For this review, take the finished solid that the model builds, in its own axes (mm). A direction names the side the tool comes from. Coordinates: 2 decimals unless noted, no trailing zeros. Write each loop counter-clockwise with the first axis right and the second up, starting at its lowest first coordinate (ties: lowest second). Pieces come first, ordered by that corner, then holes.
1) For faces 4 (the face through (15, 8, 0)), 5 (the face through (30, -6.5, -0.2)), list the 3-axis set-ups (+Z, -Z, +X, -X, +Y, -Y) from which the entire face can be reached by the end or side of a thin tool; tool diameter is ignored.
2) To check wall thickness, follow line 1 along Y through (x, z) = (12, -3.25); line 2 along Y through (x, z) = (22, -2.25); line 3 along Z through (x, y) = (14, -1). State the ranges of each line that lie inside material, in increasing order.
3) Mouldability with a two-part tool opening along Y and no side actions: class faces 1 (the face through (15, 7, 2)), 2 (the face through (15.21, -7.17, -6.97)), 3 (the face through (0, -6.5, -0.2)) as pulls with the +Y half, pulls with the -Y half, needs draft (parallel to the pull), parting line crosses it, or undercut.
4) We need section D-D on z = -9.25. Write out the cut boundary in (x, y), then the cut area to 3 significant figures.
5) We need section B-B on y = -2.5. Write out the cut boundary in (x, z), then the cut area to 3 significant figures.
6) We need section A-A on x = 6.5. Write out the cut boundary in (y, z).
7) We need section C-C on z = 4.5. Write out the cut boundary in (x, y), then the cut area to 3 significant figures.
8) Insertion check: P1, Ø2.5, axis at x = 11.5, y = 7, coming from the -Z side; P2, Ø8, axis at x = 17, z = -8.5, coming from the -Y side; P3, Ø4.5, axis at x = 18, z = 0.5, coming from the -Y side. Each pin has a flat end and moves straight along its axis. Give the tip position at first contact, or say it passes through.
from build123d import *

# Parameters (mm, degrees)
SKETCH1_W          = 30
SKETCH1_H          = 17.5
SKETCH5_R          = 6
CUT_EXTRUDE3_DEPTH = 39.890872965
SKETCH6_W          = 4
SKETCH6_H          = 4
CUT_EXTRUDE5_DEPTH = 39.890872965
SKETCH7_OUTSIDE_W  = 48.576
SKETCH7_OUTSIDE_H  = 48.576
CUT_EXTRUDE6_DEPTH = 39.890872965


with BuildPart() as part:
    # Sketch1 → Revolve1 (revolve)
    with BuildSketch(Plane.XY, mode=Mode.PRIVATE) as revolve1_sk:
        with Locations((15, 8.75)):
            Rectangle(SKETCH1_W, SKETCH1_H)
    revolve(revolve1_sk.sketch.rotate(Axis((0, 0, 0), (-1, 0, 0)), 90), axis=Axis((0, 0, 0), (-1, 0, 0)))

    # Sketch5 → Cut-Extrude3 (cut, through all)
    with BuildSketch(Plane.ZY):
        Circle(SKETCH5_R)
    extrude(amount=-CUT_EXTRUDE3_DEPTH, mode=Mode.SUBTRACT)

    # Sketch6 → Cut-Extrude5 (cut, through all)
    with BuildSketch(Plane.ZY):
        with Locations((0, 6)):
            Rectangle(SKETCH6_W, SKETCH6_H)
    extrude(amount=-CUT_EXTRUDE5_DEPTH, mode=Mode.SUBTRACT)

    # Sketch7 outside → Cut-Extrude6 (cut, through all)
    with BuildSketch(Plane(origin=(30, 0, 0), x_dir=(0, 0, -1), z_dir=(1, 0, 0))):
        Rectangle(SKETCH7_OUTSIDE_W, SKETCH7_OUTSIDE_H)
        Polygon((-14.142135624, 0), (0, -14.142135624), (14.142135624, 0), (0, 14.142135624), align=None, mode=Mode.SUBTRACT)
    extrude(amount=-CUT_EXTRUDE6_DEPTH, mode=Mode.SUBTRACT)


solid = part.part
Result:
1. face 4: +X, -X
1. face 5: +Z, -Z, +X, +Y, -Y
2. line 1: y = -10.89 to -5.04, 5.04 to 10.89
2. line 2: y = -11.89 to -5.56, 5.56 to 11.89
2. line 3: z = -13.14 to -5.92, 5.92 to 13.14
3. face 1: undercut
3. face 2: pulls with the -Y half
3. face 3: needs draft
4. outline: (0, -4.89) - (30, -4.89) - (30, 4.89) - (0, 4.89) - close
4. area: 294 mm2
5. outline: (0, -11.64) - (30, -11.64) - (30, -5.45) - (0, -5.45) - close; (0, 5.45) - (30, 5.45) - (30, 11.64) - (0, 11.64) - close
5. area: 371 mm2
6. outline: (-14.14, 0) - (0, -14.14) - (14.14, 0) - (0, 14.14) - close; hole (5.66, -2) - (8, -2) - (8, 2) - (5.66, 2) arc R6 ccw (long way) to start
7. outline: (0, -9.64) - (30, -9.64) - (30, -3.97) - (0, -3.97) - close; (0, 3.97) - (30, 3.97) - (30, 9.64) - (0, 9.64) - close
7. area: 340 mm2
8. P1: stops at z = -8.39
8. P2: stops at y = -9.64
8. P3: stops at y = -14.14
